```python
from build123d import *

# Parameters (mm, degrees)
F1_DEPTH = 38.1
F3_DEPTH = 25.4


with BuildPart() as f1:
    # F0 (on Top) → F1 (new body)
    with BuildSketch(Plane.XY):
        Polygon((-38.1, 12.7), (-38.1, 0), (-38.1, -12.7), (0, -12.7), (38.1, -12.7), (38.1, 0), (38.1, 12.7), (0, 12.7), align=None)
    extrude(amount=F1_DEPTH)

    # F2 (on face) → F3 (cut)
    with BuildSketch(Plane.XZ.offset(12.7)):
        with BuildLine():
            Line((19.05, 38.1), (-19.05, 38.1))
            ThreePointArc((-19.05, 38.1), (0, 19.05), (19.05, 38.1))
        make_face()
    extrude(amount=-F3_DEPTH, mode=Mode.SUBTRACT)


solid = f1.part
```
CAD build for the part. Positions are in the model's coordinates, mm. Coordinates: 2 decimals unless noted, no trailing zeros. Order: outer loops, then holes, each group sorted by start corner. A loop starts at its lowest first (then second) coordinate and runs counter-clockwise, first axis right, second up.
(1) Pin check, flat tip, straight feed: pin 1 Ø5 at (x, y) = (3.5, 0) entering from +Z. Stop position of the tip, or through.
Solution:
pin 1: stops at z = 20.02
(2) Saw through at C-C, the plane x = 0. Write the cut outline in (y, z).
Solution:
outline: (-12.7, 0) - (12.7, 0) - (12.7, 19.05) - (-12.7, 19.05) - close
(3) Saw through at B-B, the plane y = -9.5. Write the cut outline in (x, z), and give its area (3 significant figures).
Solution:
outline: (-38.1, 0) - (38.1, 0) - (38.1, 38.1) - (19.05, 38.1) arc R19.05 cw to (-19.05, 38.1) - (-38.1, 38.1) - close
area: 2,330 mm2
(4) Saw through at A-A, the plane z = 22. Write the cut outline in (x, y), and give its area (3 significant figures).
Solution:
outline: (-38.1, -12.7) - (-10.18, -12.7) - (-10.18, 12.7) - (-38.1, 12.7) - close; (10.18, -12.7) - (38.1, -12.7) - (38.1, 12.7) - (10.18, 12.7) - close
area: 1,420 mm2
(5) Mould opens along X. For faces 1 (the face through (38.1, 0, 19)), 2 (the face through (-38.1, 0, 19)), 3 (the face through (-0.419, -0.178, 19.055)), 4 (the face through (-29, 0, 38.1)) say: released by +X, released by -X, zero draft, split by the parting line, or undercut.
Solution:
face 1: released by +X
face 2: released by -X
face 3: undercut
face 4: zero draft
(6) Saw through at D-D, the plane x = -14. Write the cut outline in (y, z).
Solution:
outline: (-12.7, 0) - (12.7, 0) - (12.7, 25.18) - (-12.7, 25.18) - close
(7) Drill centre lines: L1, parallel to X at y = 5.5, z = 32; L2, parallel to X at y = 6.75, z = 33; L3, parallel to Z at x = -15.5, y = 6.5. Where is each one in solid material? Low to high.
Solution:
L1: x = -38.1 to -18.05, 18.05 to 38.1
L2: x = -38.1 to -18.35, 18.35 to 38.1
L3: z = 0 to 27.03
